The listing builds one solid part. Answer for the finished solid, in the listing's coordinates (mm). Face numbers are marked on the shaded views. Give positions to 0.01 mm unless a question says otherwise; leave off trailing zeros. Order: outer loops, then holes, each group sorted by start corner. A loop starts at its lowest first (then second) coordinate and runs counter-clockwise, first axis right, second up. Notation, with made-up numbers: (63, 27.5) - (99, 27.5) arc R30 ccw to (99, 62.5) - close; hole circle Ø7 at (26, -16.5). An arc over 180 degrees is marked (long way). Answer as a JSON object with one key per item and string values. Group by question number.
Q1. A cutting plane is placed at B-B, the plane y = 19. Give the vertices of the cut face in (x, z), and give its area (3 significant figures).
Q2. The mould has two halves that part along Y. Classify the marked faces 1, 2 and 3: released by +Y, released by -Y, zero draft, split by the parting line, or undercut.
Q3. A cutting plane is placed at A-A, the plane x = 34. Give the vertices of the cut face in (y, z).
Q4. A cutting plane is placed at C-C, the plane z = 21.5. Give the vertices of the cut face in (x, y), and give its area (3 significant figures).
Q5. Consider line 1 (Y direction, x = -2, z = -5); line 2 (Y direction, x = 116, z = -8); line 3 (Y direction, x = 10, z = 11). Determine where each line is inside the solid, lowest interval first.
Q6. Given pin 1 (1.8 mm diameter, centred on x = 80.5, y = -9, fed in from -Z); pin 2 (2.5 mm diameter, centred on x = 78, y = 35.5, fed in from -Z); pin 3 (1 mm diameter, centred on x = -3, y = 32, fed in from +Z), each flat-ended and moving along its own axis, determine where each tip first touches the part or whether it passes through.
Q7. A cutting plane is placed at D-D, the plane x = -20. Give the vertices of the cut face in (y, z).
from build123d import *

# Parameters (mm, degrees)
F0_R      = 30.4787407236
F1_DEPTH  = 5
F2_R      = 12.323577598
F3_DEPTH  = 3
F4_R      = 3.8165326263
F5_DEPTH  = 25
F6_R      = 12.2992477122
F7_DEPTH  = 3
F9_DEPTH  = 2
F10_W     = 133.2869231701
F10_H     = 18.6895169318
F11_DEPTH = 6
F13_DEPTH = 2
F14_W     = 133.5
F14_H     = 19
F15_DEPTH = 5
F16_R     = 4.3615258045
F17_DEPTH = 55


with BuildPart() as f1:
    # F0 (on Front) → F1 (new body)
    with BuildSketch(Plane.XZ):
        Circle(F0_R)
    extrude(amount=F1_DEPTH)

    # F2 (on face) → F3 (join)
    with BuildSketch(Plane(origin=(0, 0, 0), x_dir=(-1, 0, 0), z_dir=(0, 1, 0))):
        Circle(F2_R)
    extrude(amount=F3_DEPTH)

    # F4 (on face) → F5 (join)
    with BuildSketch(Plane(origin=(0, 3, 0), x_dir=(-1, 0, 0), z_dir=(0, 1, 0))):
        Circle(F4_R)
    extrude(amount=F5_DEPTH)

    # F6 (on face) → F7 (join)
    with BuildSketch(Plane(origin=(0, 28, 0), x_dir=(-1, 0, 0), z_dir=(0, 1, 0))):
        Circle(F6_R)
    extrude(amount=F7_DEPTH)

    # F8 (on face) → F9 (join)
    with BuildSketch(Plane.XZ.offset(5)):
        Polygon((-7.3528563089, 12.591948495), (-14.5813754343, -0.0717861064), (-7.2285191254, -12.6637346014), (7.3528563089, -12.591948495), (14.5813754343, 0.0717861064), (7.2285191254, 12.6637346014), align=None)
    extrude(amount=F9_DEPTH)

    # F10 (on face) → F11 (join)
    with BuildSketch(Plane.XZ.offset(7)):
        with Locations((66.643461585, 0)):
            Rectangle(F10_W, F10_H)
        with BuildLine():
            Line((0, -9.3447584659), (0, 9.3447584659))
            ThreePointArc((0, 9.3447584659), (-7.7820729992, 0), (0, -9.3447584659))
        make_face()
        with BuildLine():
            ThreePointArc((133.2869231701, -9.3447584659), (142.631681636, 0), (133.2869231701, 9.3447584659))
            Line((133.2869231701, 9.3447584659), (133.2869231701, -9.3447584659))
        make_face()
    extrude(amount=F11_DEPTH)

    # F12 (on face) → F13 (join)
    with BuildSketch(Plane(origin=(0, 31, 0), x_dir=(-1, 0, 0), z_dir=(0, 1, 0))):
        Polygon((7.1009739775, 12.2992477122), (-7.1009739775, 12.2992477122), (-14.2019479549, 0), (-7.1009739775, -12.2992477122), (7.1009739775, -12.2992477122), (14.2019479549, 0), align=None)
    extrude(amount=F13_DEPTH)

    # F14 (on face) → F15 (join)
    with BuildSketch(Plane(origin=(0, 33, 0), x_dir=(-1, 0, 0), z_dir=(0, 1, 0))):
        with Locations((-66.75, 0)):
            Rectangle(F14_W, F14_H)
        with BuildLine():
            Line((0, 9.5), (0, -9.5))
            ThreePointArc((0, -9.5), (7.6147800585, 0), (0, 9.5))
        make_face()
        with BuildLine():
            ThreePointArc((-133.5, 9.5), (-143, 0), (-133.5, -9.5))
            Line((-133.5, -9.5), (-133.5, 9.5))
        make_face()
    extrude(amount=F15_DEPTH)

    # F16 (on face) → F17 (cut)
    with BuildSketch(Plane.XZ.offset(13)):
        with Locations((133.2869231701, 0)):
            Circle(F16_R)
    extrude(amount=-F17_DEPTH, mode=Mode.SUBTRACT)


solid = f1.part
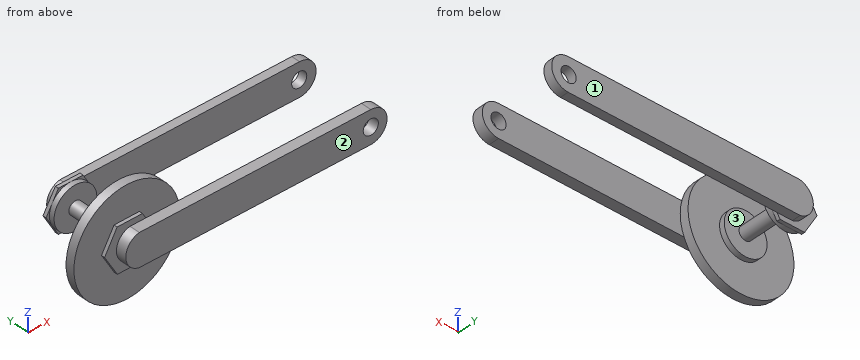
Reply:
{
 "1": {"outline": "circle Ø7.63 at (0, 0)", "area": "45.8 mm^2"},
 "2": {"face 1": "released by +Y", "face 2": "released by -Y", "face 3": "undercut"},
 "3": {"outline": "(-13, -9.34) - (-7, -9.34) - (-7, 9.34) - (-13, 9.34) - close; (33, -9.5) - (38, -9.5) - (38, 9.5) - (33, 9.5) - close"},
 "4": {"outline": "(-21.6, -5) - (21.6, -5) - (21.6, 0) - (-21.6, 0) - close", "area": "216 mm^2"},
 "5": {"line 1": "y = -13 to 3, 28 to 38", "line 2": "y = -13 to -7, 33 to 38", "line 3": "y = -5 to 0"},
 "6": {"pin 1": "stops at z = -9.34", "pin 2": "stops at z = -9.5", "pin 3": "stops at z = 12.3"},
 "7": {"outline": "(-5, -23) - (0, -23) - (0, 23) - (-5, 23) - close"}
}
